Work out the finished part from the listing and answer in its coordinate system (mm). A direction names the side the tool comes from. Coordinates: 2 decimals unless noted, no trailing zeros. Loops run counter-clockwise (first coordinate to the right, second up) from the corner with the lowest first, then second, coordinate; pieces in that order, holes last. Notation, with made-up numbers: (-11, 68) -> (40, 68) arc R28 cw to (40, 91) -> close; hole circle Ø9 at (-6.5, 64). An arc over 180 degrees is marked (long way). Answer as CSV lines item,"result".
Autodesk Inventor part; units mm, degrees
ref_plane "YZ Plane" through (0, 0, 0) normal (1, 0, 0) x (0, 1, 0)
ref_plane "XZ Plane" through (0, 0, 0) normal (0, 1, 0) x (-1, 0, 0)
ref_plane "XY Plane" through (0, 0, 0) normal (0, 0, 1) x (1, 0, 0)
sketch "Эскиз1" plane through (0, 0, 0) normal (0, 0, 1) x (1, 0, 0)
  line L0 (-37, -47) -> (37, -47)
  line L1 (37, -47) -> (37, 47)
  line L2 (37, 47) -> (-37, 47)
  line L3 (-37, 47) -> (-37, -47)
  line L4 (-35, -44) -> (-35, 44)
  line L5 (34, -45) -> (-34, -45)
  line L6 (35, 44) -> (35, -44)
  line L7 (-34, 45) -> (34, 45)
  point P0 (0, 0)
  dimension "d0" = 2
  dimension "d1" = 2
  dimension "d2" = 2
  dimension "d3" = 2
extrude "Выдавливание1" add sketch "Эскиз1" along normal blind 2
sketch "Эскиз2" plane through (0, 0, 2) normal (0, 0, 1) x (1, 0, 0)
  line L0 (-39, -49) -> (39, -49)
  line L1 (39, -49) -> (39, 49)
  line L2 (39, 49) -> (-39, 49)
  line L3 (-39, 49) -> (-39, -49)
  line L4 (-37, 47) -> (-37, -47)
  line L5 (-37, -47) -> (37, -47)
  line L6 (37, -47) -> (37, 47)
  line L7 (37, 47) -> (-37, 47)
  point P0 (0, 0)
  dimension "d6" = 2
  dimension "d7" = 2
  dimension "d8" = 2
  dimension "d9" = 2
extrude "Выдавливание2" add sketch "Эскиз2" against normal blind 25
sketch "Эскиз3" plane through (-39, -49, 2) normal (-1, 0, 0) x (0, 0, 1)
  line L0 (-3.5, 69) -> (-3.5, 78)
  line L1 (-3.5, 69) -> (-14.5, 69)
  line L2 (-14.5, 78) -> (-14.5, 69)
  line L3 (-3.5, 78) -> (-14.5, 78)
  point P0 (-2, 49)
extrude "Выдавливание3" cut sketch "Эскиз3" against normal blind 25
sketch "Эскиз4" plane through (-39, -49, 2) normal (-1, 0, 0) x (0, 0, 1)
  line L0 (-3.5, 69) -> (-3.5, 78)
  line L1 (-3.5, 78) -> (-14.5, 78)
  line L2 (-14.5, 69) -> (-14.5, 78)
  line L3 (-3.5, 69) -> (-14.5, 69)
  line L4 (-15.0649, 68.3908) -> (-2.9071, 68.3908)
  line L5 (-2.9071, 68.3908) -> (-2.9071, 78.6857)
  line L6 (-2.9071, 78.6857) -> (-15.0649, 78.6857)
  line L7 (-15.0649, 78.6857) -> (-15.0649, 68.3908)
  point P0 (-2, 49)
extrude "Выдавливание4" cut sketch "Эскиз4" against normal blind 25
sketch "Эскиз5" plane through (-39, -49, 2) normal (0, -1, 0) x (1, 0, 0)
  line L0 (19, -3.5) -> (6, -3.5)
  line L1 (19, -3.5) -> (19, -19.5)
  line L2 (6, -19.5) -> (19, -19.5)
  line L3 (6, -3.5) -> (6, -19.5)
  line L4 (65, -3.5) -> (38, -3.5)
  line L5 (65, -3.5) -> (65, -9.5)
  line L6 (54, -9.5) -> (65, -9.5)
  line L7 (54, -9.5) -> (54, -16.5)
  line L8 (38, -16.5) -> (54, -16.5)
  line L9 (38, -3.5) -> (38, -16.5)
  line L10 (2, -25) -> (76, -25)
  line L11 (6, -3.5) -> (54, -3.5)
  line L12 (54, -3.5) -> (54, -25)
  line L13 (54, -25) -> (6, -25)
  line L14 (6, -25) -> (6, -3.5)
  line L15 (54, -25) -> (6, -25)
  line L16 (6, -25) -> (6, -2.7247)
  line L17 (6, -2.7247) -> (54, -2.7247)
  line L18 (54, -2.7247) -> (54, -25)
  point P0 (39, -2)
  point P1 (6, -25)
extrude "Выдавливание5" cut sketch "Эскиз5" against normal blind 25 contours L1 L2 L3 L0 | L11 L9 L8 L12 L10 L14 L2 L1 | L4 L12 L7 L8 L9
sketch "Эскиз6" plane through (39, -49, 2) normal (1, 0, 0) x (0, 0, -1)
  arc A0 (8.5, 75) -> (8.5, 81) centre (8.5, 78) ccw
  arc A1 (6.5, 81) -> (6.5, 75) centre (6.5, 78) ccw
  line L0 (6.5, 75) -> (8.5, 75)
  arc A2 (8.5, 75) -> (8.5, 81) centre (8.5, 78) ccw
  line L1 (6.5, 81) -> (8.5, 81)
  line L2 (25, 0) -> (25, 98)
  line L3 (3.5, 81) -> (25, 81)
  line L4 (25, 81) -> (25, 75)
  line L5 (25, 75) -> (3.5, 75)
  line L6 (3.5, 75) -> (3.5, 81)
  point P0 (2, 49)
  point P1 (6.5, 75)
  point P2 (8.5, 75)
  point P3 (8.5, 81)
  point P4 (6.5, 81)
extrude "Выдавливание6" cut sketch "Эскиз6" against normal blind 25
sketch "Эскиз7" plane through (-39, -49, 2) normal (-1, 0, 0) x (0, 0, 1)
  point P0 (-2, 49)
sketch "Эскиз8" plane through (-39, -49, 2) normal (-1, 0, 0) x (0, 0, 1)
  line L0 (-15.0649, 68.3908) -> (-15.0649, 78.6857)
  line L1 (-15.0649, 78.6857) -> (-15.0649, 68.3908)
  line L2 (-15.0649, 68.3908) -> (-19.0649, 68.3908)
  line L3 (-19.0649, 68.3908) -> (-19.0649, 78.6857)
  line L4 (-19.0649, 78.6857) -> (-15.0649, 78.6857)
  line L5 (-15.0649, 78.6857) -> (-15.0649, 68.3908)
  point P0 (-2, 49)
  dimension "d20" = 4
extrude "Выдавливание7" cut sketch "Эскиз8" against normal blind 10
equation "\"d7\" = d6"
equation "\"d8\" = d7"
equation "\"d9\" = d7"
properties part number "btn"
(1) A cutting plane is placed at D-D, the plane y = 3. Write down the section's boundary in (x, z), and give its area (3 significant figures).
Computed values:
outline,"(-39, -23) -> (-37, -23) -> (-37, 0) -> (37, 0) -> (37, -23) -> (39, -23) -> (39, 2) -> (-39, 2) -> close"
area,"248 mm2"
(2) A cutting plane is placed at B-B, the plane z = -20.5. Write down the section's boundary in (x, y).
Computed values:
outline,"(-39, -49) -> (-33, -49) -> (-33, -47) -> (-37, -47) -> (-37, 47) -> (37, 47) -> (37, 32) -> (39, 32) -> (39, 49) -> (-39, 49) -> close; (15, -49) -> (39, -49) -> (39, 26) -> (37, 26) -> (37, -47) -> (15, -47) -> close"
(3) Which of the six approach directions +Z, -Z, +X, -X, +Y, -Y give full straight-line access (tool end or side, diameter ignored) to faces 5 (the face through (-37, 1, -11)), 6 (the face through (38, 29, -1.5)), 7 (the face through (-38, 24, -17.065))?
Computed values:
face 5,"-Z"
face 6,"-Z, +X"
face 7,"-X"
(4) For a pull along Z with two mould halves and no side action, classify faces 1 (the face through (-38, 19.391, -9)), 2 (the face through (-38, 29.686, -9)), 3 (the face through (39, -1, -10)), 4 (the face through (38, -22, -23)) as pulls with the +Z half, pulls with the -Z half, needs draft (parallel to the pull), parting line crosses it, or undercut.
Computed values:
face 1,"undercut"
face 2,"undercut"
face 3,"needs draft"
face 4,"pulls with the -Z half"
(5) A cutting plane is placed at C-C, the plane x = 18. Write down the section's boundary in (y, z), and give its area (3 significant figures).
Computed values:
outline,"(-49, -23) -> (-47, -23) -> (-47, 0) -> (47, 0) -> (47, -23) -> (49, -23) -> (49, 2) -> (-49, 2) -> close"
area,"288 mm2"
(6) Flat-ended cylindrical pins translate along their axes: pin 1 Ø1 at (x, z) = (-25.5, -16) entering from -Y; pin 2 Ø6 at (x, y) = (18, 29.5) entering from -Z; pin 3 Ø1 at (x, y) = (1.5, -48.5) entering from -Z. Find the tip coordinate at first contact, or state that the pin passes through.
Computed values:
pin 1,"y = 47"
pin 2,"z = 0"
pin 3,"z = -1.5"
(7) Consider line 1 along Y through (x, z) = (35, -1.5); line 2 along X through (y, z) = (-32.5, -16.25); line 3 along Z through (x, y) = (29, -34). Determine where each line is inside the solid, lowest interval first.
Computed values:
line 1,"-49 to -47, 47 to 49"
line 2,"-39 to -37, 37 to 39"
line 3,"0 to 2"
(8) A cutting plane is placed at A-A, the plane z = -12.75. Write down the section's boundary in (x, y).
Computed values:
outline,"(-39, -49) -> (-33, -49) -> (-33, -47) -> (-37, -47) -> (-37, 19.39) -> (-39, 19.39) -> close; (-39, 29.69) -> (-37, 29.69) -> (-37, 47) -> (37, 47) -> (37, 32) -> (39, 32) -> (39, 49) -> (-39, 49) -> close; (15, -49) -> (39, -49) -> (39, 26) -> (37, 26) -> (37, -47) -> (15, -47) -> close"
